Autodesk Inventor part; units mm, degrees
ref_plane "YZ Plane" through (0, 0, 0) normal (1, 0, 0) x (0, 1, 0)
ref_plane "XZ Plane" through (0, 0, 0) normal (0, 1, 0) x (-1, 0, 0)
ref_plane "XY Plane" through (0, 0, 0) normal (0, 0, 1) x (1, 0, 0)
sketch "Sketch1" plane through (0, 0, 0) normal (0, 0, 1) x (1, 0, 0)
  line L0 (0, 0) -> (20, 0)
  line L1 (20, 0) -> (20, -20)
  line L2 (20, -20) -> (0, -20)
  line L3 (0, -20) -> (0, 0)
  dimension "d0" = 20
  dimension "d1" = 20
extrude "Extrusion1" add sketch "Sketch1" along normal blind 850
sketch "Sketch2" plane through (0, 0, 850) normal (0, 0, 1) x (1, 0, 0)
  line L0 (1, -1) -> (19, -1)
  line L1 (19, -1) -> (19, -19)
  line L2 (19, -19) -> (1, -19)
  line L3 (1, -19) -> (1, -1)
  line L4 (0, 0) -> (0, -20)
  line L5 (20, 0) -> (0, 0)
  dimension "d4" = 1
  dimension "d5" = 1
  dimension "d6" = 18
  dimension "d7" = 18
extrude "Extrusion2" cut sketch "Sketch2" against normal through all
properties part number "profil_handle"
For this review, take the finished solid that the model builds, in its own axes (mm). A direction names the side the tool comes from. Round coordinates to 2 decimals unless told otherwise and drop trailing zeros. Order: outer loops, then holes, each group sorted by start corner. A loop starts at its lowest first (then second) coordinate and runs counter-clockwise, first axis right, second up. Notation, with made-up numbers: (41, 30.5) -> (87, 30.5) arc R7 ccw to (87, 43.5) -> close; hole circle Ø6 at (-10, 32.5). An arc over 180 degrees is marked (long way). Put each result on its own line as item: value.
Q1. Machinability: for faces 1 (the flat face through (9.2, -19.6, 850)), 2 (the flat face through (10, -19, 431)), which of the approach directions +Z, -Z, +X, -X, +Y, -Y give a long, thin tool a straight path to every point of the face, cutting with its end or side? Answer none if there is none.
Check result:
face 1: +Z, +X, -X, +Y, -Y
face 2: +Z, -Z
Q2. Mouldability with a two-part tool opening along X and no side actions: class faces 3 (the flat face through (0, -10, 419)), 4 (the flat face through (10, 0, 419)), 5 (the flat face through (1, -10, 431)) as pulls with the +X half, pulls with the -X half, needs draft (parallel to the pull), parting line crosses it, or undercut.
Check result:
face 3: pulls with the -X half
face 4: needs draft
face 5: undercut
Q3. Add section C-C on z = 581. Write out the cut boundary in (x, y).
Check result:
outline: (0, -20) -> (20, -20) -> (20, 0) -> (0, 0) -> close; hole (1, -19) -> (19, -19) -> (19, -1) -> (1, -1) -> close
Q4. Add section B-B on x = 5.25. Write out the cut boundary in (y, z).
Check result:
outline: (-20, 0) -> (-19, 0) -> (-19, 850) -> (-20, 850) -> close; (-1, 0) -> (0, 0) -> (0, 850) -> (-1, 850) -> close
Q5. Insertion check: pin 1 Ø8 at (x, y) = (5.5, -8) entering from +Z. The pin has a flat end and moves straight along its axis. Give the tip position at first contact, or say it passes through.
Check result:
pin 1: through
Q6. For probe 1 along X at (y, z) = (-3, 506.5); probe 2 along Y at (x, z) = (14.75, 494), list the stretches that pass through material, from the lowest coordinate up. Write a range as [from, to].
Check result:
probe 1: [0, 1], [19, 20]
probe 2: [-20, -19], [-1, 0]
Q7. Add section A-A on y = -11. Write out the cut boundary in (x, z), plus the area to 3 significant figures.
Check result:
outline: (0, 0) -> (1, 0) -> (1, 850) -> (0, 850) -> close; (19, 0) -> (20, 0) -> (20, 850) -> (19, 850) -> close
area: 1,700 mm2
